Autodesk Inventor part; units mm, degrees
ref_plane "YZ Plane" through (0, 0, 0) normal (1, 0, 0) x (0, 1, 0)
ref_plane "XZ Plane" through (0, 0, 0) normal (0, 1, 0) x (-1, 0, 0)
ref_plane "XY Plane" through (0, 0, 0) normal (0, 0, 1) x (1, 0, 0)
sketch "Sketch1" plane through (0, 0, 0) normal (1, 0, 0) x (0, 1, 0)
  point P0 (0, 0)
sketch "Sketch2" plane through (0, 0, 0) normal (1, 0, 0) x (0, 1, 0)
  line L0 (0, 0) -> (0, -431.8)
  line L1 (0, -431.8) -> (88.9, -431.8)
  line L2 (88.9, -431.8) -> (88.9, -88.9)
  line L3 (88.9, -88.9) -> (749.3, -88.9)
  line L4 (749.3, -88.9) -> (749.3, -431.8)
  line L5 (749.3, -431.8) -> (838.2, -431.8)
  line L6 (838.2, -431.8) -> (838.2, 0)
  line L7 (838.2, 0) -> (0, 0)
  dimension "d0" = 660.4
  dimension "d1" = 342.9
  dimension "d2" = 342.9
  dimension "d3" = 88.9
  dimension "d4" = 88.9
  dimension "d5" = 88.9
extrude "Extrusion1" add sketch "Sketch2" along normal blind 127
fillet "Fillet1" radius 25.4 14 edges at (127, 419.1, 0) (0, 419.1, 0) (63.5, 838.2, 0) (127, 838.2, -215.9) (0, 838.2, -215.9) (63.5, 0, 0) (127, 0, -215.9) (127, 44.45, -431.8) (127, 793.75, -431.8) (63.5, 838.2, -431.8) (0, 793.75, -431.8) (0, 0, -215.9) (0, 44.45, -431.8) (63.5, 0, -431.8)
sketch "Sketch3" plane through (0, 88.9, -88.9) normal (0, 0, -1) x (-1, 0, 0)
  line L0 (0, 0) -> (-127, 0)
  line L1 (-63.5, 0) -> (-63.5, 660.4)
  line L2 (-25.4, 660.4) -> (-101.6, 660.4)
  line L3 (-63.5, 0) -> (-63.5, 254)
  line L4 (-63.5, 254) -> (-63.5, 406.4)
  line L5 (-63.5, 406.4) -> (-63.5, 660.4)
  line L6 (-63.5, 254) -> (-63.5, 292.1)
  line L7 (-63.5, 406.4) -> (-63.5, 368.3)
  circle A0 centre (-63.5, 292.1) radius 2.54
  circle A1 centre (-63.5, 368.3) radius 2.54
  line L8 (0, 0) -> (0, 660.4)
  line L9 (0, 406.4) -> (0, 368.3)
  line L10 (-127, 0) -> (-127, 660.4)
  line L11 (-60.96, 292.1) -> (-66.04, 292.1)
  line L12 (-63.5, 254) -> (-127, 254)
  line L13 (-127, 254) -> (-127, 292.1)
  line L14 (-127, 292.1) -> (-88.9, 292.1)
  line L15 (-127, 368.3) -> (-88.9, 368.3)
  line L16 (0, 292.1) -> (-38.1, 292.1)
  line L17 (0, 368.3) -> (-38.1, 368.3)
  circle A2 centre (-88.9, 292.1) radius 2.54
  circle A3 centre (-88.9, 368.3) radius 2.54
  circle A4 centre (-38.1, 368.3) radius 2.54
  circle A5 centre (-38.1, 292.1) radius 2.54
  point P0 (0, -88.9)
  dimension "d9" = 254
  dimension "d10" = 152.4
  dimension "d23" = 38.1
  dimension "d24" = 38.1
  dimension "d25" = 38.1
extrude "Extrusion2" cut sketch "Sketch3" against normal blind 3.175 contours A1 L1 | L1 A1 | A0 L11 L1 | L1 L11 A0 | L11 A0 L1 | L1 A0 L11
sketch "Sketch4" plane through (0, 88.9, -88.9) normal (0, 0, -1) x (-1, 0, 0)
  line L0 (0, 0) -> (-127, 0)
  line L1 (0, 0) -> (0, 292.1)
  line L2 (0, 0) -> (0, 660.4)
  line L3 (0, 292.1) -> (0, 368.3)
  line L4 (0, 292.1) -> (-38.1, 292.1)
  line L5 (0, 368.3) -> (-38.1, 368.3)
  line L6 (-127, 0) -> (-127, 660.4)
  line L7 (-127, 292.1) -> (-88.9, 292.1)
  line L8 (-127, 368.3) -> (-88.9, 368.3)
  circle A0 centre (-88.9, 292.1) radius 2.54
  circle A1 centre (-38.1, 292.1) radius 2.54
  circle A2 centre (-38.1, 368.3) radius 2.54
  circle A3 centre (-88.9, 368.3) radius 2.54
  point P0 (0, -88.9)
  dimension "d26" = 292.1
  dimension "d27" = 76.2
  dimension "d28" = 38.1
  dimension "d30" = 38.1
  dimension "d31" = 5.08
  dimension "d50" = 38.1
  dimension "d51" = 38.1
extrude "Extrusion3" cut sketch "Sketch4" against normal blind 3.175
sketch "Sketch5" plane through (0, 749.3, -88.9) normal (0, -1, 0) x (1, 0, 0)
  line L0 (0, 0) -> (0, -317.5)
  line L1 (0, -152.3238) -> (87.3252, -152.3238)
  line L2 (25.4, -342.9) -> (101.6, -342.9)
  line L3 (127, 0) -> (127, -317.5)
  line L4 (127, -152.3238) -> (39.6748, -152.3238)
  circle A0 centre (87.3252, -152.3238) radius 2.54
  circle A1 centre (39.6748, -152.3238) radius 2.54
  line L5 (87.3252, -152.3238) -> (87.3252, -101.5238)
  line L6 (39.6748, -152.3238) -> (39.6748, -101.5238)
  circle A2 centre (39.6748, -101.5238) radius 2.54
  circle A3 centre (87.3252, -101.5238) radius 2.54
  line L7 (87.3252, -101.5238) -> (87.3252, 0)
  point P0 (0, 88.9)
  dimension "d34" = 87.3252
  dimension "d36" = 87.3252
  dimension "d37" = 5.08
  dimension "d40" = 50.8
extrude "Extrusion5" cut sketch "Sketch5" against normal blind 3.175
sketch "Sketch6" plane through (0, 88.9, -88.9) normal (0, 1, 0) x (1, 0, 0)
  arc A0 (127, 317.5) -> (101.6, 342.9) centre (101.6, 317.5) ccw
  line L0 (127, 317.5) -> (127, 0)
  line L1 (101.6, 317.5) -> (25.4, 317.5)
  line L2 (101.6, 317.5) -> (127, 317.5)
  line L3 (101.6, -63.5) -> (101.6, 317.5)
  line L4 (101.6, 317.5) -> (101.6, 133.35)
  line L5 (101.6, 133.35) -> (101.6, 95.25)
  line L6 (25.4, 133.35) -> (25.4, 95.25)
  circle A1 centre (101.6, 133.35) radius 2.54
  circle A2 centre (101.6, 95.25) radius 2.54
  circle A3 centre (25.4, 95.25) radius 2.54
  circle A4 centre (25.4, 133.35) radius 2.54
  line L7 (101.6, -88.9) -> (25.4, -88.9)
  line L8 (101.6, 317.5) -> (101.6, -88.9)
  line L9 (25.4, 95.25) -> (25.4, 0)
  point P0 (0, -88.9)
  dimension "d46" = 38.1
  dimension "d47" = 5.08
extrude "Extrusion6" cut sketch "Sketch6" against normal blind 3.175
properties part number "Bumper"
Could you check a few things on this model? Use its own coordinates, in mm. Give positions to 0.01 mm unless a question says otherwise; leave off trailing zeros. Order: outer loops, then holes, each group sorted by start corner. A loop starts at its lowest first (then second) coordinate and runs counter-clockwise, first axis right, second up. Notation, with made-up numbers: (2, 39.5) -> (12, 39.5) arc R23 ccw to (12, 53.5) -> close; hole circle Ø11 at (13.25, 60). An arc over 180 degrees is marked (long way). Return JSON: item names as keys, results as strings.
1. For pin 1 Ø6.5 at (x, y) = (63.5, 457.2) entering from -Z; pin 2 Ø1.5 at (x, y) = (39, 458.5) entering from -Z (3 decimals), each with a flat end and sliding along its axis, tell me the tip position at first contact or that it passes through.
Answer list:
{"pin 1": "stops at z = -88.9", "pin 2": "stops at z = -85.725"}
2. Imagine slicing it at A-A on z = -284.5. List the corners of the cut face in (x, y) for me, then the cut area to 3 significant figures.
Answer list:
{"outline": "(0, 25.4) arc R25.4 ccw to (25.4, 0) -> (101.6, 0) arc R25.4 ccw to (127, 25.4) -> (127, 88.9) -> (0, 88.9) -> close; (0, 749.3) -> (127, 749.3) -> (127, 812.8) arc R25.4 ccw to (101.6, 838.2) -> (25.4, 838.2) arc R25.4 ccw to (0, 812.8) -> close", "area": "22,000 mm2"}
3. Imagine slicing it at B-B on y = 112. List the corners of the cut face in (x, z) for me, then the cut area to 3 significant figures.
Answer list:
{"outline": "(0, -88.9) -> (127, -88.9) -> (127, -25.4) arc R25.4 ccw to (101.6, 0) -> (25.4, 0) arc R25.4 ccw to (0, -25.4) -> close", "area": "11,000 mm2"}
4. I need wall thicknesses on line 1 (Z direction, x = 101.6, y = 87.75); line 2 (X direction, y = 87.7, z = -222.25); line 3 (Y direction, x = 88.9, z = -87.65). Which ranges of each line are inside material? Lowest first, please. Write a range as from..to.
Answer list:
{"line 1": "z = -431.8..-224.79, -219.71..-186.69, -181.61..0", "line 2": "x = 0..22.86, 27.94..99.06, 104.14..127", "line 3": "y = 0..378.46, 383.54..454.66, 459.74..838.2"}
